Verification items for the finished model (mm, model axes). A direction names the side the tool comes from. Coordinates: 2 decimals unless noted, no trailing zeros. Write each loop counter-clockwise with the first axis right and the second up, starting at its lowest first coordinate (ties: lowest second). Pieces come first, ordered by that corner, then holes. Notation, with made-up numbers: (52.25, -23.5) - (69.25, -23.5) arc R21 cw to (69.25, -15.5) - close; hole circle Ø6 at (-33.5, 50). An arc over 180 degrees is marked (long way). Answer as CSV lines item,"result". Start each with the question number.
```python
from build123d import *

# Parameters (mm, degrees)
SKETCH1_W                  = 31.75
SKETCH1_H                  = 26.9748
SKETCH1_R                  = 2.1336
BASE_FLANGE1_DEPTH         = 3.175
SKETCHED_START             = 9.335343098
SKETCHED_BEND1_OUTLINE_W   = 31.75
SKETCHED_BEND1_OUTLINE_H   = 3.175
SKETCHED_BEND1_DEPTH       = 11.543456902
SKETCHED_START_2           = 6.160343098
SKETCHED_BEND1_2_OUTLINE_W = 31.75
SKETCHED_BEND1_2_OUTLINE_H = 12.815143098
SKETCHED_BEND1_2_OUTLINE_R = 2.1336
SKETCHED_BEND1_2_DEPTH     = 2.71893284
SKETCHED_START_3           = 5.017343098
SKETCHED_BEND1_3_OUTLINE_W = 31.75
SKETCHED_BEND1_3_OUTLINE_H = 12.815143098
SKETCHED_BEND1_3_OUTLINE_R = 2.1336
SKETCHED_BEND1_3_DEPTH     = 4.318
SKETCHED_START_4           = -15.875
SKETCHED_BEND1_4_DEPTH     = 31.75
CHAMFER1_SIZE              = 0.381
FILLET1_R                  = 0.635


with BuildPart() as part:
    # Base-Flange1: sheet metal written as solids
    # Sketch1 → Base-Flange1 (new body)
    with BuildSketch(Plane.XY):
        with Locations((0, 7.3914)):
            Rectangle(SKETCH1_W, SKETCH1_H)
        with Locations((9.525, 0)):
            Circle(SKETCH1_R, mode=Mode.SUBTRACT)
        with Locations((-9.525, 0)):
            Circle(SKETCH1_R, mode=Mode.SUBTRACT)
        with Locations((9.525, 16.9164)):
            Circle(SKETCH1_R, mode=Mode.SUBTRACT)
        with Locations((-9.525, 16.9164)):
            Circle(SKETCH1_R, mode=Mode.SUBTRACT)
    extrude(amount=BASE_FLANGE1_DEPTH)

    # Sketched Bend1: read off the stored shape, not the designer's step
    # Sketched Bend1 outline → Sketched Bend1 (cut)
    with BuildSketch(Plane(origin=(0, 0, 0), x_dir=(1, 0, 0), z_dir=(0, 1, 0)).offset(SKETCHED_START)):
        with Locations((0, -1.5875)):
            Rectangle(SKETCHED_BEND1_OUTLINE_W, SKETCHED_BEND1_OUTLINE_H)
    extrude(amount=SKETCHED_BEND1_DEPTH, mode=Mode.SUBTRACT)

    # Sketched Bend1 2 outline → Sketched Bend1 2 (add)
    with BuildSketch(Plane(origin=(0, 0, 0), x_dir=(1, 0, 0), z_dir=(0, 1, 0)).offset(SKETCHED_START_2)):
        with Locations((0, -9.582571549)):
            Rectangle(SKETCHED_BEND1_2_OUTLINE_W, SKETCHED_BEND1_2_OUTLINE_H)
        with Locations((-9.525, -12.027743098)):
            Circle(SKETCHED_BEND1_2_OUTLINE_R, mode=Mode.SUBTRACT)
        with Locations((9.525, -12.027743098)):
            Circle(SKETCHED_BEND1_2_OUTLINE_R, mode=Mode.SUBTRACT)
    extrude(amount=SKETCHED_BEND1_2_DEPTH)

    # Sketched Bend1 3 outline → Sketched Bend1 3 (add)
    with BuildSketch(Plane(origin=(0, 0, 0), x_dir=(1, 0, 0), z_dir=(0, 1, 0)).offset(SKETCHED_START_3)):
        with Locations((0, -9.582571549)):
            Rectangle(SKETCHED_BEND1_3_OUTLINE_W, SKETCHED_BEND1_3_OUTLINE_H)
        with Locations((-9.525, -12.027743098)):
            Circle(SKETCHED_BEND1_3_OUTLINE_R, mode=Mode.SUBTRACT)
        with Locations((9.525, -12.027743098)):
            Circle(SKETCHED_BEND1_3_OUTLINE_R, mode=Mode.SUBTRACT)
    extrude(amount=SKETCHED_BEND1_3_DEPTH)

    # Sketched Bend1 4 outline → Sketched Bend1 4 (cut)
    with BuildSketch(Plane.YZ.offset(SKETCHED_START_4)):
        with BuildLine():
            Line((6.160343098, 4.318), (6.160343098, 15.990143098))
            Line((6.160343098, 15.990143098), (5.017343098, 15.990143098))
            Line((5.017343098, 15.990143098), (5.017343098, 3.175))
            ThreePointArc((5.017343098, 3.175), (5.825566149, 3.509776949), (6.160343098, 4.318))
        make_face()
        with BuildLine():
            Line((9.335343098, 0), (9.335343098, 4.318))
            ThreePointArc((9.335343098, 4.318), (8.070630179, 1.264712919), (5.017343098, 0))
            Line((5.017343098, 0), (9.335343098, 0))
        make_face()
    extrude(amount=SKETCHED_BEND1_4_DEPTH, mode=Mode.SUBTRACT)

    # Chamfer1
    chamfer1_edges = [part.edges().sort_by_distance(p)[0] for p in [
        (7.3914, 9.335343098, 12.027743098),
        (7.3914, 6.160343098, 12.027743098),
        (-11.6586, 9.335343098, 12.027743098),
        (-11.6586, 6.160343098, 12.027743098),
    ]]
    chamfer(chamfer1_edges, length=CHAMFER1_SIZE)

    # Fillet1
    fillet1_edges = [part.edges().sort_by_distance(p)[0] for p in [
        (-15.875, -6.096, 1.5875),
        (15.875, -6.096, 1.5875),
        (-15.875, 7.747843098, 15.990143098),
        (15.875, 7.747843098, 15.990143098),
    ]]
    fillet(fillet1_edges, radius=FILLET1_R)


solid = part.part
```
1. Access from +Z, -Z, +X, -X, +Y, -Y to the whole of each face (thin tool, end or side, straight path). Record for faces 1 (the face through (0, 8, 15.99)), 2 (the face through (0, 0, 3.175)).
2. Depth check by flat-ended pin: P1, Ø3.5, axis at x = 5, z = 9, coming from the -Y side. Enter the tip coordinate at first touch or a pass-through.
3. Cross-section at A-A (y = 0). Record the cut outline in (x, z) (3 decimals).
4. Cross-section at C-C (z = 9). Record the cut outline in (x, y) (3 decimals).
5. Cross-section at D-D (y = 2.75). Record the cut outline in (x, z) (3 decimals), and give its area (3 significant figures).
6. Draft check along X on faces 3 (the face through (-11.218, -1.298, 1.565)), 4 (the face through (-15.875, 7, 6)), 5 (the face through (15.875, 7, 6)), 6 (the face through (0, 6.16, 10)). Enter one of: pulls with the +X half, pulls with the -X half, needs draft (parallel to the pull), parting line crosses it, or undercut.
7. Cross-section at B-B (x = -4.5). Record the cut outline in (y, z) (3 decimals), and give its area (3 significant figures).
8. Scan lines: line 1 along X through (y, z) = (-0.25, 1.75) (3 decimals); line 2 along Z through (x, y) = (11, 2) (3 decimals); line 3 along Y through (x, z) = (-1.5, 7.25). Record each from-to range of solid material in increasing order. Write a range as from..to.
Completed:
1,face 1,"+Z, +X, -X, +Y, -Y"
1,face 2,"+Z, +X, -X, -Y"
2,P1,"stops at y = 6.16"
3,outline,"(-15.875, 0) - (-11.659, 0) - (-11.659, 3.175) - (-15.875, 3.175) - close; (-7.391, 0) - (7.391, 0) - (7.391, 3.175) - (-7.391, 3.175) - close; (11.659, 0) - (15.875, 0) - (15.875, 3.175) - (11.659, 3.175) - close"
4,outline,"(-15.875, 6.16) - (15.875, 6.16) - (15.875, 9.335) - (-15.875, 9.335) - close"
5,outline,"(-15.875, 0) - (15.875, 0) - (15.875, 3.175) - (-15.875, 3.175) - close"
5,area,"101 mm2"
6,face 3,"undercut"
6,face 4,"pulls with the -X half"
6,face 5,"pulls with the +X half"
6,face 6,"needs draft"
7,outline,"(-6.096, 0) - (5.017, 0) arc R4.318 ccw to (9.335, 4.318) - (9.335, 15.99) - (6.16, 15.99) - (6.16, 4.318) arc R1.143 cw to (5.017, 3.175) - (-6.096, 3.175) - close"
7,area,"86.0 mm2"
8,line 1,"x = -15.875..-11.644, -7.406..7.406, 11.644..15.875"
8,line 2,"z = 0..3.175"
8,line 3,"y = 6.16..9.34"
